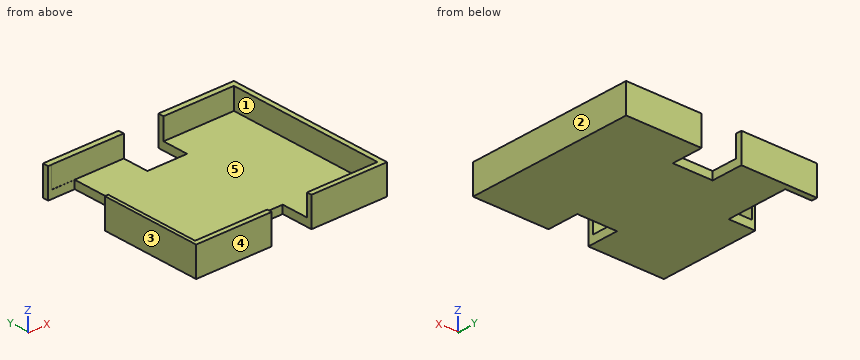
from build123d import *

# Parameters (mm, degrees)
SKETCH_W        = 36
SKETCH_H        = 32
PAD_DEPTH       = 5.5
SKETCH001_W     = 34.4
SKETCH001_H     = 30
POCKET_DEPTH    = 4
SKETCH002_W     = 11.815998
SKETCH002_H     = 6.205499
POCKET001_DEPTH = 5
SKETCH003_W     = 7.5
SKETCH003_H     = 9.005811
POCKET002_DEPTH = 6
SKETCH004_W     = 7.5
SKETCH004_H     = 11.328424
POCKET003_DEPTH = 6


with BuildPart() as part:
    # Sketch → Pad (new body)
    with BuildSketch(Plane.XY):
        with Locations((18, 16)):
            Rectangle(SKETCH_W, SKETCH_H)
    extrude(amount=PAD_DEPTH)

    # Sketch001 (on Face6 of Pad) → Pocket (cut)
    with BuildSketch(Plane.XY.offset(5.5)):
        with Locations((17.841014, 15.929226)):
            Rectangle(SKETCH001_W, SKETCH001_H)
    extrude(amount=-POCKET_DEPTH, mode=Mode.SUBTRACT)

    # Sketch002 (on Face2 of Pocket) → Pocket001 (cut)
    with BuildSketch(Plane(origin=(0, 0, 0), x_dir=(0, -1, 0), z_dir=(-1, 0, 0))):
        with Locations((-24.999628, 2.678109)):
            Rectangle(SKETCH002_W, SKETCH002_H)
    extrude(amount=-POCKET001_DEPTH, mode=Mode.SUBTRACT)

    # Sketch003 (on Face1 of Pocket001) → Pocket002 (cut)
    with BuildSketch(Plane.XZ):
        with Locations((18, 2.765324)):
            Rectangle(SKETCH003_W, SKETCH003_H)
    extrude(amount=-POCKET002_DEPTH, mode=Mode.SUBTRACT)

    # Sketch004 (on Face7 of Pocket001) → Pocket003 (cut)
    with BuildSketch(Plane(origin=(0, 32, 0), x_dir=(-1, 0, 0), z_dir=(0, 1, 0))):
        with Locations((-18.017854, 3.606522)):
            Rectangle(SKETCH004_W, SKETCH004_H)
    extrude(amount=-POCKET003_DEPTH, mode=Mode.SUBTRACT)


solid = part.part
Design review of the part built by this model. Coordinates are the model's own, in mm. Face numbers are marked on the shaded views. A direction names the side the tool comes from. Round coordinates to 2 decimals unless told otherwise and drop trailing zeros. Write each loop counter-clockwise with the first axis right and the second up, starting at its lowest first coordinate (ties: lowest second). Pieces come first, ordered by that corner, then holes. Notation, with made-up numbers: (34.5, -3.5) -> (62.5, -3.5) arc R9 ccw to (62.5, 0.5) -> close; hole circle Ø7 at (61, 75.5). An arc over 180 degrees is marked (long way). One line per item, written item: value. Start each with the question number.
Q1. Add section D-D (y = 30.5). Give the boundary of the cut face in (x, z).
Q2. Add section C-C (z = 4.5). State how many separate pieces and enclosed holes the cut face has, then the cut area to 3 significant figures.
Q3. Tool access review of the marked faces 4 and 5: name each direction out of +Z, -Z, +X, -X, +Y, -Y from which nothing blocks a thin tool from reaching the whole face with its end or side.
Q4. The part is to be moulded in two halves that separate along X. For the marked faces 1, 2 and 3, say which applies: pulls with the +X half, pulls with the -X half, needs draft (parallel to the pull), parting line crosses it, or undercut.
Q5. To check wall thickness, follow probe 1 along X at (y, z) = (30.5, 0.95); probe 2 along Y at (x, z) = (22, 2.4); probe 3 along X at (y, z) = (13, 2.1). State the ranges of each line that lie inside material, in increasing order.
Q6. Add section A-A (y = 5). Give the boundary of the cut face in (x, z).
Q7. Insertion check: P1, Ø12, axis at x = 15.5, y = 16.5, coming from the +Z side; P2, Ø3, axis at y = 25.5, z = 4.5, coming from the -X side; P3, Ø3, axis at y = 29, z = 1.5, coming from the -X side. Each pin has a flat end and moves straight along its axis. Give the tip position at first contact, or say it passes through.
Response:
1. outline: (5, 0) -> (14.27, 0) -> (14.27, 1.5) -> (5, 1.5) -> close; (21.77, 0) -> (36, 0) -> (36, 5.5) -> (35.04, 5.5) -> (35.04, 1.5) -> (21.77, 1.5) -> close
2. separate pieces: 3
2. enclosed holes: 0
2. area: 97.4 mm^2
3. face 4: +Z, -Z, +X, -X, -Y
3. face 5: +Z
4. face 1: undercut
4. face 2: pulls with the +X half
4. face 3: pulls with the -X half
5. probe 1: x = 5 to 14.27, 21.77 to 36
5. probe 2: y = 0 to 0.93, 30.93 to 32
5. probe 3: x = 0 to 0.64, 35.04 to 36
6. outline: (0, 0) -> (14.25, 0) -> (14.25, 1.5) -> (0.64, 1.5) -> (0.64, 5.5) -> (0, 5.5) -> close; (21.75, 0) -> (36, 0) -> (36, 5.5) -> (35.04, 5.5) -> (35.04, 1.5) -> (21.75, 1.5) -> close
7. P1: stops at z = 1.5
7. P2: stops at x = 35.04
7. P3: stops at x = 5
